```python
from build123d import *

# Parameters (mm, degrees)
ESQUISSE1_W                  = 60
ESQUISSE1_H                  = 18
BOSS_EXTRU_1_DEPTH           = 25
ESQUISSE2_W                  = 40
ESQUISSE2_H                  = 20
ENL_V_MAT_EXTRU_1_DEPTH      = 30
CONG_1_R                     = 5
ESQUISSE3_R                  = 2.15
ENL_V_MAT_EXTRU_2_DEPTH      = 30
ENL_V_MAT_EXTRU_3_DEPTH      = 66.620118866
ENL_V_MAT_EXTRU_3_DEPTH_BACK = 80
ESQUISSE4_W                  = 5
ESQUISSE4_H                  = 2


with BuildPart() as part:
    # Esquisse1 → Boss.-Extru.1 (new body)
    with BuildSketch(Plane.XY):
        Rectangle(ESQUISSE1_W, ESQUISSE1_H)
    extrude(amount=BOSS_EXTRU_1_DEPTH)

    # Esquisse2 → Enlèv. mat.-Extru.1 (cut)
    with BuildSketch(Plane.XZ.offset(9)):
        with Locations((0, 12.5)):
            Rectangle(ESQUISSE2_W, ESQUISSE2_H)
    extrude(amount=-ENL_V_MAT_EXTRU_1_DEPTH, mode=Mode.SUBTRACT)

    # Congé1
    cong_1_edges = [part.edges().sort_by_distance(p)[0] for p in [
        (-30, 0, 25),
        (30, 0, 25),
        (-30, 0, 0),
        (30, 0, 0),
    ]]
    fillet(cong_1_edges, radius=CONG_1_R)

    # Esquisse3 → Enlèv. mat.-Extru.2 (cut)
    with BuildSketch(Plane(origin=(0, -9, 0), x_dir=(-1, 0, 0), z_dir=(0, -1, 0))):
        with Locations(Location((23.9, -17.6, 0), (0, 0, 90))):
            Circle(ESQUISSE3_R)
        with Locations(Location((23.9, -7.4, 0), (0, 0, 90))):
            Circle(ESQUISSE3_R)
        with Locations(Location((-23.9, -7.4, 0), (0, 0, 90))):
            Circle(ESQUISSE3_R)
        with Locations(Location((-23.9, -17.6, 0), (0, 0, 90))):
            Circle(ESQUISSE3_R)
    extrude(amount=-ENL_V_MAT_EXTRU_2_DEPTH, mode=Mode.SUBTRACT)

    # Esquisse4 → Enlèv. mat.-Extru.3 (cut, two sides: drawn at the far end of the back side and taken through both)
    with BuildSketch(Plane.ZY.offset(30).offset(-ENL_V_MAT_EXTRU_3_DEPTH_BACK)):
        with Locations((7.4, 2)):
            Rectangle(ESQUISSE4_W, ESQUISSE4_H)
        with Locations((17.6, 2)):
            Rectangle(ESQUISSE4_W, ESQUISSE4_H)
    extrude(amount=ENL_V_MAT_EXTRU_3_DEPTH + ENL_V_MAT_EXTRU_3_DEPTH_BACK, mode=Mode.SUBTRACT)


solid = part.part
```
Could you check a few things on this model? Use its own coordinates, in mm. A direction names the side the tool comes from. Round coordinates to 2 decimals unless told otherwise and drop trailing zeros. Loops run counter-clockwise (first coordinate to the right, second up) from the corner with the lowest first, then second, coordinate; pieces in that order, holes last.
Q1. Please list where these lines run through material, in increasing order: L1, parallel to X at y = -6, z = 7.4; L2, parallel to Z at x = 17, y = 0.75; L3, parallel to X at y = -3, z = 11.75.
Q2. Thinking about a two-plate mould opening in X: for faces 1 (the flat face through (0, 0, 2.5)), 2 (the flat face through (-25, 2, 20.1)), 3 (the flat face through (-30, 0, 12)), which applies, pulls with the +X half, pulls with the -X half, needs draft (parallel to the pull), parting line crosses it, or undercut?
Q3. I want a section at B-B (y = -0.75). Write out the boundary of the cut face in (x, z).
Q4. On a 3-axis mill with a long thin cutter (end or side, diameter ignored), from which of +Z, -Z, +X, -X, +Y, -Y can I reach the whole of each face in a straight line? I mean faces 4 (the flat face through (0, 0, 22.5)), 5 (the flat face through (-7, 9, 23)), 6 (the flat face through (-25, 2, 4.9)). Say none if no direction works.
Q5. I want a section at C-C (x = -11.5). Write out the boundary of the cut face in (y, z), and give its area (3 significant figures).
Q6. I want a section at A-A (z = 7.4). Give the number of separate pieces and of enclosed holes in the cut face, and give its area (3 significant figures).
Q7. For P1, Ø0.6, axis at x = -27, y = 1.5, coming from the -Z side, with a flat end and sliding along its axis, tell me the tip position at first contact or that it passes through.
Q8. I want a section at D-D (x = 23.9). Write out the boundary of the cut face in (y, z), and give its area (3 significant figures).
Answer below:
1. L1: x = -30 to -26.05, -21.75 to -20, 20 to 21.75, 26.05 to 30
1. L2: z = 0 to 2.5, 22.5 to 25
1. L3: x = -30 to -20, 20 to 30
2. face 1: undercut
2. face 2: needs draft
2. face 3: pulls with the -X half
3. outline: (-30, 5) arc R5 ccw to (-25, 0) - (25, 0) arc R5 ccw to (30, 5) - (30, 20) arc R5 ccw to (25, 25) - (-25, 25) arc R5 ccw to (-30, 20) - close; hole circle Ø4.3 at (-23.9, 7.4); hole circle Ø4.3 at (-23.9, 17.6); hole (-20, 2.5) - (20, 2.5) - (20, 22.5) - (-20, 22.5) - close; hole circle Ø4.3 at (23.9, 7.4); hole circle Ø4.3 at (23.9, 17.6)
4. face 4: +Y, -Y
4. face 5: +Z, -Z, +X, -X, +Y
4. face 6: +X, -X
5. outline: (-9, 0) - (9, 0) - (9, 2.5) - (-9, 2.5) - close; (-9, 22.5) - (9, 22.5) - (9, 25) - (-9, 25) - close
5. area: 90.0 mm2
6. separate pieces: 8
6. enclosed holes: 0
6. area: 182 mm2
7. P1: stops at z = 0.3
8. outline: (-9, 0) - (9, 0) - (9, 5.25) - (3, 5.25) - (3, 4.9) - (1, 4.9) - (1, 5.25) - (-9, 5.25) - close; (-9, 9.55) - (1, 9.55) - (1, 9.9) - (3, 9.9) - (3, 9.55) - (9, 9.55) - (9, 15.45) - (3, 15.45) - (3, 15.1) - (1, 15.1) - (1, 15.45) - (-9, 15.45) - close; (-9, 19.75) - (1, 19.75) - (1, 20.1) - (3, 20.1) - (3, 19.75) - (9, 19.75) - (9, 25) - (-9, 25) - close
8. area: 292 mm2
